Check sheet for the modelled part. Datum: model origin and axes. Units: mm. A direction names the side the tool comes from. Round coordinates to 2 decimals unless told otherwise and drop trailing zeros. Loops run counter-clockwise (first coordinate to the right, second up) from the corner with the lowest first, then second, coordinate; pieces in that order, holes last. Notation, with made-up numbers: M -2,76.25 L 18,76.25 A31 cw 18,113.25 Z; hole C 37,54 d2. An arc over 180 degrees is marked long. Write item = value, one per line. Start each with the question number.
(1) Cross-section at C-C on x = 4. Record the boundary of the cut face in (y, z).
(2) Cross-section at A-A on y = -12.75. Record the boundary of the cut face in (x, z), plus the area to 3 significant figures.
(3) Cross-section at D-D on x = 22. Record the boundary of the cut face in (y, z), plus the area to 3 significant figures.
(4) Go/stop test with flat-tipped pins: P1, Ø1.5, axis at x = 3.5, z = 30.5, coming from the +Y side; P2, Ø6.5, axis at x = 22, y = -10, coming from the +Z side; P3, Ø9, axis at y = -5, z = 41.5, coming from the +X side; P4, Ø4, axis at y = -14, z = 56.5, coming from the -X side. Record where each tip stops, or that it passes through.
(5) Set-up check for faces 1 (the face through (3, -9, 34)), 2 (the face through (0, -7, 47)), 3 (the face through (18, -7, 47)): record each of +Z, -Z, +X, -X, +Y, -Y from which the full face is reachable in a straight line by a thin tool's end or side.
(6) Mould release check, pull along Y, two halves, no side actions. Record for faces 4 (the face through (-1, -9, 13)), 5 (the face through (12, 0, 34)), 6 (the face through (9, -15, 34)): pulls with the +Y half, pulls with the -Y half, needs draft (parallel to the pull), parting line crosses it, or undercut.
(7) Scan lines: L1, parallel to X at y = -9.75, z = 23; L2, parallel to Y at x = 12, z = 4.5; L3, parallel to X at y = -12.5, z = 55. Record each from-to range of solid material in increasing order. Write a range as from..to.
(8) Cross-section at B-B on z = 21. Record the boundary of the cut face in (x, y).
from build123d import *

# Parameters (mm, degrees)
SKETCH_1_W          = 18
SKETCH_1_H          = 18
SKETCH_1_W_2        = 12
SKETCH_1_H_2        = 12
EXTRUDE_1_DEPTH     = 68
SKETCH_2_R          = 1.05
CUT_EXTRUDE_1_DEPTH = 32
SKETCH_3_W          = 26
SKETCH_3_H          = 18
EXTRUDE_2_DEPTH     = 5.8
SKETCH_4_W          = 26
SKETCH_4_H          = 18
EXTRUDE_3_DEPTH     = 1
SKETCH_5_R          = 1.05
CUT_EXTRUDE_2_DEPTH = 41


with BuildPart() as part:
    # 草图1 → 凸台-拉伸1 (new body)
    with BuildSketch(Plane.XY):
        with Locations((9, -9)):
            Rectangle(SKETCH_1_W, SKETCH_1_H)
        with Locations((9, -9)):
            Rectangle(SKETCH_1_W_2, SKETCH_1_H_2, mode=Mode.SUBTRACT)
    extrude(amount=EXTRUDE_1_DEPTH)

    # 草图2 → 切除-拉伸1 (cut)
    with BuildSketch(Plane(origin=(18, 0, 0), x_dir=(0, 0, -1), z_dir=(1, 0, 0))):
        with Locations((-62, -9)):
            Circle(SKETCH_2_R)
        with Locations((-47, -9)):
            Circle(SKETCH_2_R)
        with Locations((-32, -9)):
            Circle(SKETCH_2_R)
        with Locations((-6, -9)):
            Circle(SKETCH_2_R)
        with Locations((-21, -9)):
            Circle(SKETCH_2_R)
    extrude(amount=-CUT_EXTRUDE_1_DEPTH, mode=Mode.SUBTRACT)

    # 草图3 → 凸台-拉伸2 (add)
    with BuildSketch(Plane(origin=(18, 0, 0), x_dir=(0, 0, -1), z_dir=(1, 0, 0))):
        with Locations((-13, -9)):
            Rectangle(SKETCH_3_W, SKETCH_3_H)
    extrude(amount=EXTRUDE_2_DEPTH)

    # 草图4 → 凸台-拉伸3 (add)
    with BuildSketch(Plane.ZY):
        with Locations((13, -9)):
            Rectangle(SKETCH_4_W, SKETCH_4_H)
    extrude(amount=EXTRUDE_3_DEPTH)

    # 草图5 → 切除-拉伸2 (cut)
    with BuildSketch(Plane(origin=(23.8, 0, 0), x_dir=(0, 0, -1), z_dir=(1, 0, 0))):
        with Locations((-6, -9)):
            Circle(SKETCH_5_R)
        with Locations((-21, -9)):
            Circle(SKETCH_5_R)
    extrude(amount=-CUT_EXTRUDE_2_DEPTH, mode=Mode.SUBTRACT)


solid = part.part
Result:
q1.outline = M -18,0 L -15,0 L -15,68 L -18,68 Z; M -3,0 L 0,0 L 0,68 L -3,68 Z
q2.outline = M -1,0 L 3,0 L 3,68 L 0,68 L 0,26 L -1,26 Z; M 15,0 L 23.8,0 L 23.8,26 L 18,26 L 18,68 L 15,68 Z
q2.area = 585 mm^2
q3.outline = M -18,0 L 0,0 L 0,26 L -18,26 Z; hole C -9,6 d2.1; hole C -9,21 d2.1
q3.area = 461 mm^2
q4.P1 = 0
q4.P2 = 26
q4.P3 = 18
q4.P4 = 0
q5.face_1 = +Z, -Z
q5.face_2 = +Z, -X, +Y, -Y
q5.face_3 = +Z, +X, +Y, -Y
q6.face_4 = needs draft
q6.face_5 = pulls with the +Y half
q6.face_6 = undercut
q7.L1 = -1..3, 15..23.8
q7.L2 = -18..-15, -3..0
q7.L3 = 0..3, 15..18
q8.outline = M -1,-18 L 23.8,-18 L 23.8,-10.05 L 15,-10.05 L 15,-15 L 3,-15 L 3,-10.05 L -1,-10.05 Z; M -1,-7.95 L 3,-7.95 L 3,-3 L 15,-3 L 15,-7.95 L 23.8,-7.95 L 23.8,0 L -1,0 Z
